The figure shows three views and two pictorial views of one solid part (mm, origin at its lowest corner). Answer the questions. A direction names the side the tool comes from. Give positions to 0.01 mm unless a question says otherwise; leave off trailing zeros. Write each loop counter-clockwise with the first axis right and the second up, starting at its lowest first coordinate (ties: lowest second). Pieces come first, ordered by that corner, then holes. Notation, with made-up numbers: (-13.75, 5.25) - (39.25, 5.25) arc R25 cw to (39.25, 27.25) - close; hole circle Ø1 at (35.25, 61). An arc over 180 degrees is marked (long way). Write each question's results on one line, items separated by ' | '. Start each with the question number.
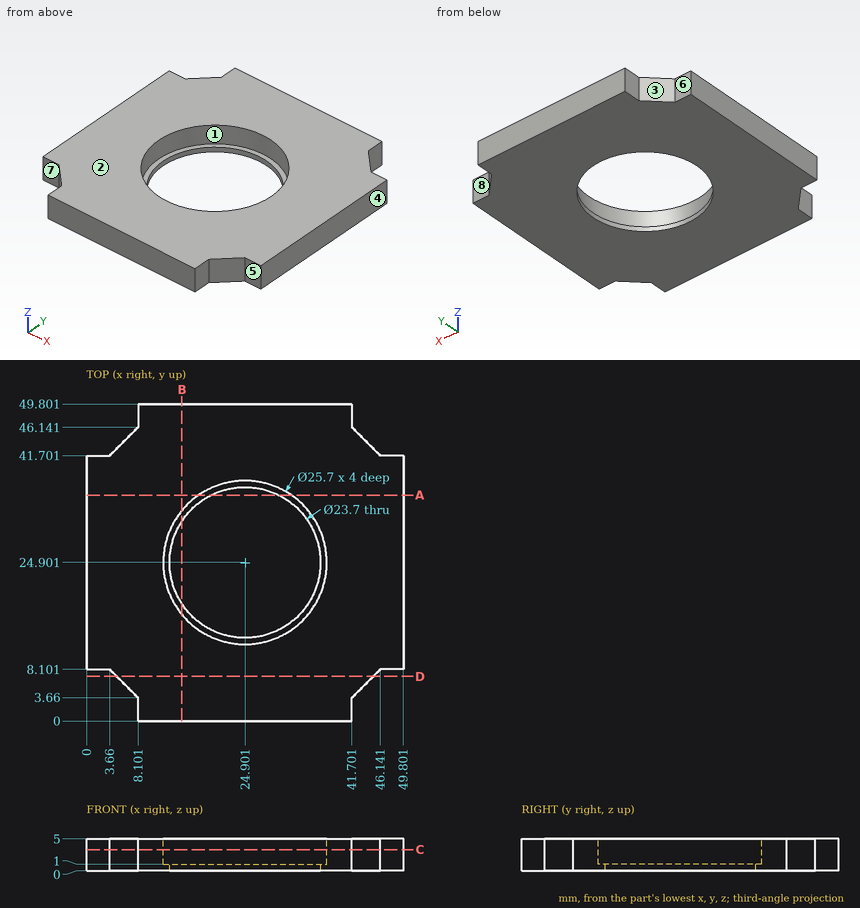
Q1. The mould has two halves that part along X. Classify the marked faces 1, 2, 3 and 4: pulls with the +X half, pulls with the -X half, needs draft (parallel to the pull), parting line crosses it, or undercut.
Q2. Consider L1, parallel to Y at x = 3.5, z = 2.4; L2, parallel to X at y = 25.5, z = 2.85 (1 decimal); L3, parallel to X at y = 16, z = 3.4. Determine where each line is inside the solid, lowest interval first.
Q3. A tool of negligible diameter and unlimited length cuts with its end or side. For the marked faces 5, 6, 7 and 8, from which of +Z, -Z, +X, -X, +Y, -Y can it reach the whole face along a straight path? Write none if from no direction.
Q4. A cutting plane is placed at A-A, the plane y = 35.5. Write down the section's boundary in (x, z) (1 decimal), and give its area (3 significant figures).
Q5. A cutting plane is placed at D-D, the plane y = 7. Write down the section's boundary in (x, z), and give its area (3 significant figures).
Q6. A cutting plane is placed at B-B, the plane x = 15. Write down the section's boundary in (y, z).
Q7. Given pin 1 (3 mm diameter, centred on y = 1, z = 1.5, fed in from +X); pin 2 (3 mm diameter, centred on x = 1.5, z = 2.5, fed in from +Y); pin 3 (1.8 mm diameter, centred on x = 1.5, z = 3, fed in from -Y), each flat-ended and moving along its own axis, determine where each tip first touches the part or whether it passes through.
Q8. A cutting plane is placed at C-C, the plane z = 3.35. Write down the section's boundary in (x, y), and give its area (3 significant figures).
Result:
1) face 1: undercut | face 2: needs draft | face 3: pulls with the -X half | face 4: pulls with the +X half
2) L1: y = 8.1 to 41.7 | L2: x = 0 to 12.1, 37.7 to 49.8 | L3: x = 0 to 15.63, 34.17 to 49.8
3) face 5: +Z, -Z, +X, -Y | face 6: +Z, -Z, -X, +Y | face 7: +Z, -Z, -X, -Y | face 8: +Z, -Z, +X, +Y
4) outline: (0, 0) - (19.6, 0) - (19.6, 1) - (17.6, 1) - (17.6, 5) - (0, 5) - close; (30.2, 0) - (49.8, 0) - (49.8, 5) - (32.2, 5) - (32.2, 1) - (30.2, 1) - close | area: 180 mm2
5) outline: (4.76, 0) - (45.04, 0) - (45.04, 5) - (4.76, 5) - close | area: 201 mm2
6) outline: (0, 0) - (18.39, 0) - (18.39, 1) - (16.71, 1) - (16.71, 5) - (0, 5) - close; (31.41, 0) - (49.8, 0) - (49.8, 5) - (33.09, 5) - (33.09, 1) - (31.41, 1) - close
7) pin 1: stops at x = 41.7 | pin 2: stops at y = 41.7 | pin 3: stops at y = 8.1
8) outline: (0, 8.1) - (3.66, 8.1) - (8.1, 3.66) - (8.1, 0) - (41.7, 0) - (41.7, 3.66) - (46.14, 8.1) - (49.8, 8.1) - (49.8, 41.7) - (46.14, 41.7) - (41.7, 46.14) - (41.7, 49.8) - (8.1, 49.8) - (8.1, 46.14) - (3.66, 41.7) - (0, 41.7) - close; hole circle Ø25.7 at (24.9, 24.9) | area: 1,740 mm2
